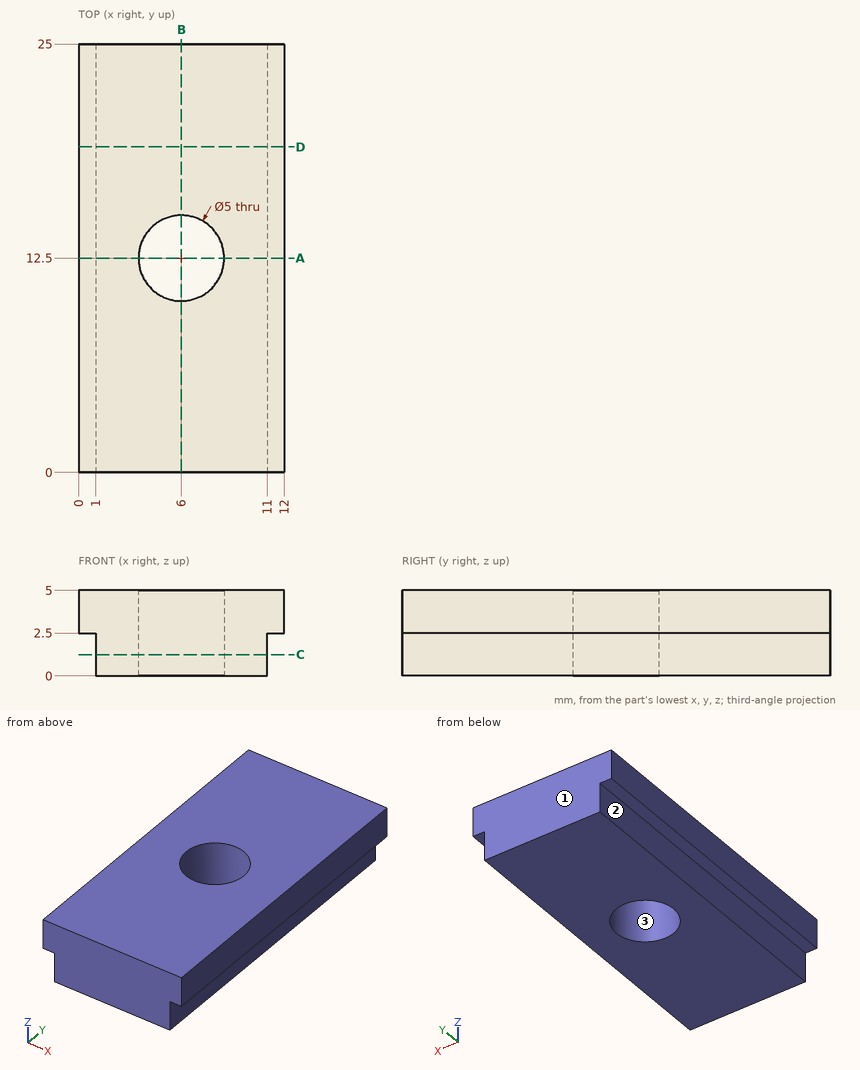
Verification items for this drawing (mm, ordinates from the low corner). Coordinates: 2 decimals unless noted, no trailing zeros. Write each loop counter-clockwise with the first axis right and the second up, starting at its lowest first coordinate (ties: lowest second). Pieces come first, ordered by that corner, then holes. Notation, with made-up numbers: (85, 76.25) -> (93, 76.25) arc R13 cw to (93, 97.25) -> close; hole circle Ø4 at (54.25, -29). An arc over 180 degrees is marked (long way). Use CSV: the item, a comma, the result in double quotes. Start each with the question number.
Item 1: Cross-section at B-B, the plane x = 6. Record the cut outline in (y, z).
Item 2: Thickness scan on line 1 (Y direction, x = 6, z = 1); line 2 (X direction, y = 24.25, z = 1.5); line 3 (X direction, y = 11, z = 2.2). Record the ranges inside material, lowest first.
Item 3: Mould release check, pull along X, two halves, no side actions. Record for the marked faces 1, 2 and 3: released by +X, released by -X, zero draft, split by the parting line, or undercut.
Item 4: Cross-section at D-D, the plane y = 19. Record the cut outline in (x, z).
Item 5: Cross-section at C-C, the plane z = 1.25. Record the cut outline in (x, y), plus the area to 3 significant figures.
Item 6: Cross-section at A-A, the plane y = 12.5. Record the cut outline in (x, z).
Item 7: Depth check by flat-ended pin: pin 1 Ø1.2 at (y, z) = (12.5, 1) entering from +X; pin 2 Ø6 at (x, y) = (6, 12.5) entering from -Z; pin 3 Ø2 at (y, z) = (11, 1) entering from -X. Enter the tip coordinate at first touch or a pass-through.
Answers:
1,outline,"(0, 0) -> (10, 0) -> (10, 5) -> (0, 5) -> close; (15, 0) -> (25, 0) -> (25, 5) -> (15, 5) -> close"
2,line 1,"0 to 10, 15 to 25"
2,line 2,"1 to 11"
2,line 3,"1 to 4, 8 to 11"
3,face 1,"zero draft"
3,face 2,"released by -X"
3,face 3,"undercut"
4,outline,"(0, 2.5) -> (1, 2.5) -> (1, 0) -> (11, 0) -> (11, 2.5) -> (12, 2.5) -> (12, 5) -> (0, 5) -> close"
5,outline,"(1, 0) -> (11, 0) -> (11, 25) -> (1, 25) -> close; hole circle Ø5 at (6, 12.5)"
5,area,"230 mm^2"
6,outline,"(0, 2.5) -> (1, 2.5) -> (1, 0) -> (3.5, 0) -> (3.5, 5) -> (0, 5) -> close; (8.5, 0) -> (11, 0) -> (11, 2.5) -> (12, 2.5) -> (12, 5) -> (8.5, 5) -> close"
7,pin 1,"x = 11"
7,pin 2,"z = 0"
7,pin 3,"x = 1"
